```python
from build123d import *

# Parameters (mm, degrees)
F1_DEPTH = 500
F3_T     = -2
F5_DEPTH = 2


with BuildPart() as f1:
    # F0 (on Top) → F1 (new body)
    with BuildSketch(Plane.XY):
        with BuildLine():
            Line((-450, 0), (0, 0))
            Line((0, 0), (0, 450))
            ThreePointArc((0, 450), (-318.198052, 318.198052), (-450, 0))
        make_face()
    extrude(amount=F1_DEPTH)

    # F2: F1 across plane


with BuildPart() as f1_1:
    add(f1.part)
    add(f1.part.mirror(Plane.YZ))

    # F3
    f3_openings = [f1_1.faces().sort_by_distance(p)[0] for p in [
        (0, 0, 250),
    ]]
    offset(amount=F3_T, openings=f3_openings)

    # F4 (on face) → F5 (cut, through all)
    with BuildSketch(Plane.XY.offset(2)):
        with BuildLine():
            ThreePointArc((448, 0), (0, 448), (-448, 0))
            Line((-448, 0), (448, 0))
        make_face()
    extrude(amount=-F5_DEPTH, mode=Mode.SUBTRACT)


solid = f1_1.part
```
The model under review builds one solid part; all positions refer to its coordinate system, in mm. Give positions to 0.01 mm unless a question says otherwise; leave off trailing zeros. Write each loop counter-clockwise with the first axis right and the second up, starting at its lowest first coordinate (ties: lowest second). Pieces come first, ordered by that corner, then holes.
(1) Consider section D-D, the plane x = 243. Give the boundary of the cut face in (y, z).
(2) To check wall thickness, follow L1, parallel to Z at x = -54, y = 72; L2, parallel to X at y = 344.5, z = 204; L3, parallel to X at y = 375, z = 52.5. State the ranges of each line that lie inside material, in increasing order.
(3) Consider section B-B, the plane y = 142.5. Give the boundary of the cut face in (x, z).
(4) Consider section A-A, the plane x = -148. Give the boundary of the cut face in (y, z), and give its area (3 significant figures).
(5) For P1, Ø12, axis at x = 304, z = 258, coming from the +Y side; P2, Ø2, axis at x = -227, z = 320, coming from the -Y side; P3, Ø2, axis at x = 107, y = 62, coming from the -Z side, all flat-tipped, find the tip position at first contact; note any pin that passes through.
(6) Consider section C-C, the plane z = 345. Give the boundary of the cut face in (x, y).
(7) The part is to be moulded in two halves that separate along X. For faces 1 (the flat face through (6, 177, 498)), 2 (the flat face through (6, 178, 500)), say which applies: released by +X, released by -X, zero draft, split by the parting line, or undercut.
Returned:
1. outline: (0, 498) - (376.37, 498) - (376.37, 0) - (378.75, 0) - (378.75, 500) - (0, 500) - close
2. L1: z = 498 to 500
2. L2: x = -289.52 to -286.4, 286.4 to 289.52
2. L3: x = -248.75 to -245.11, 245.11 to 248.75
3. outline: (-426.84, 0) - (-424.73, 0) - (-424.73, 498) - (424.73, 498) - (424.73, 0) - (426.84, 0) - (426.84, 500) - (-426.84, 500) - close
4. outline: (0, 498) - (422.85, 498) - (422.85, 0) - (424.97, 0) - (424.97, 500) - (0, 500) - close
4. area: 1,900 mm2
5. P1: stops at y = 337.19
5. P2: stops at y = 385.64
5. P3: stops at z = 498
6. outline: (-450, 0) - (-448, 0) arc R448 cw to (0, 448) arc R448 cw to (448, 0) - (450, 0) arc R450 ccw to (0, 450) arc R450 ccw to start
7. face 1: undercut
7. face 2: zero draft
